from build123d import *

# Parameters (mm, degrees)
F0_W      = 76.2
F0_H      = 76.2
F1_DEPTH  = 76.2
F2_W      = 50.8
F2_H      = 50.8
F3_DEPTH  = 50.8
F4_W      = 7.2508919984
F4_H      = 10.1156122983
F5_DEPTH  = 12.7
F6_R      = 5.08
F7_W      = 8.5941962898
F7_H      = 18.2563401759
F8_DEPTH  = 2.54
F10_W     = 29.7498870641
F10_H     = 30.6668374687
F11_DEPTH = 2.54
F12_R     = 5.08
F13_W     = 35.6998704374
F13_H     = 3.7890225649
F14_DEPTH = 25.4
F16_W     = 13.0332894623
F16_H     = 16.8449506164
F17_DEPTH = 2.54
F18_DEPTH = 2.54
F19_DEPTH = 2.54


with BuildPart() as f1:
    # F0 (on Top) → F1 (new body)
    with BuildSketch(Plane.XY):
        with Locations((-38.1, 38.1)):
            Rectangle(F0_W, F0_H)
    extrude(amount=F1_DEPTH)

    # F2 (on face) → F3 (join)
    with BuildSketch(Plane.YZ):
        with Locations((42.4093476772, 25.4)):
            Rectangle(F2_W, F2_H)
    extrude(amount=F3_DEPTH)

    # F4 (on face) → F5 (join)
    with BuildSketch(Plane.XY.offset(50.8)):
        with Locations((22.3073018715, 41.2539299577)):
            Rectangle(F4_W, F4_H)
    extrude(amount=F5_DEPTH)

    # F6
    f6_edges = [f1.edges().sort_by_distance(p)[0] for p in [
        (22.307302, 36.196124, 63.5),
    ]]
    fillet(f6_edges, radius=F6_R)

    # F7 (on face) → F8 (join)
    with BuildSketch(Plane.XZ):
        with Locations((-42.4338337034, 9.1281700879)):
            Rectangle(F7_W, F7_H)
    extrude(amount=F8_DEPTH)

    # F10 (on face) → F11 (join)
    with BuildSketch(Plane.XZ.offset(-17.0093476772)):
        with Locations((22.7058520541, 15.3334187344)):
            Rectangle(F10_W, F10_H)
    extrude(amount=F11_DEPTH)

    # F12
    f12_edges = [f1.edges().sort_by_distance(p)[0] for p in [
        (-38.1, 0, 76.2),
        (0, 38.1, 76.2),
        (-38.1, 76.2, 76.2),
        (-76.2, 38.1, 76.2),
    ]]
    fillet(f12_edges, radius=F12_R)

    # F13 (on face) → F14 (join)
    with BuildSketch(Plane.XZ):
        with Locations((-39.2985325307, 46.8699112535)):
            Rectangle(F13_W, F13_H)
    extrude(amount=F14_DEPTH)

    # F16 (on face) → F17 (join)
    with BuildSketch(Plane.XZ):
        with Locations((-39.2985325307, 57.1868978441)):
            Rectangle(F16_W, F16_H)
    extrude(amount=F17_DEPTH)

    # F15 (on face) → F18 (join)
    with BuildSketch(Plane.XY.offset(48.7644225359)):
        Polygon((-57.1484677494, -18.2180759441), (-52.4711199105, -25.4), (-48.1553934515, -25.4), (-57.1484677494, -11.2543340924), align=None)
    extrude(amount=F18_DEPTH)

    # F19 (add): a face of the model
    f19_faces = [f1.faces().sort_by_distance(p)[0] for p in [
        (-38.1323314504, -12.5401378745, 48.7644225359),
    ]]
    extrude(f19_faces, amount=F19_DEPTH)


solid = f1.part
For this review, take the finished solid that the model builds, in its own axes (mm). A direction names the side the tool comes from. Round coordinates to 2 decimals unless told otherwise and drop trailing zeros. Order: outer loops, then holes, each group sorted by start corner. A loop starts at its lowest first (then second) coordinate and runs counter-clockwise, first axis right, second up. Notation, with made-up numbers: (86.25, 31) -> (100.25, 31) arc R18 cw to (100.25, 38) -> close; hole circle Ø6 at (-24.75, 10). An arc over 180 degrees is marked (long way). Write item = value, one per line. Start each with the question number.
1) To check wall thickness, follow line 1 (Y direction, x = 14.5, z = 37); line 2 (X direction, y = 55, z = 71); line 3 (Z direction, x = 20.5, y = 61). State the ranges of each line that lie inside material, in increasing order. Write a range as from..to.
2) Insertion check: pin 1 (0.8 mm diameter, centred on y = -0.5, z = 10.5, fed in from +X); pin 2 (1 mm diameter, centred on x = -39.5, z = 39, fed in from -Y); pin 3 (5 mm diameter, centred on x = -55.5, y = -22.5, fed in from +Z); pin 4 (2 mm diameter, centred on x = 27, z = 62.5, fed in from +Y). Each pin has a flat end and moves straight along its axis. Give the tip position at first contact, or say it passes through.
3) Take a section at C-C on z = 23. State the section outline as (x, y) points, plus the area to 3 significant figures.
4) Take a section at D-D on y = 55.5. State the section outline as (x, z) points, plus the area to 3 significant figures.
5) Take a section at A-A on z = 56. State the section outline as (x, y) points, plus the area to 3 significant figures.
6) Tool access review of faces 1 (the face through (-57.148, -13, 48)), 2 (the face through (-42, -2.54, 9)), 3 (the face through (22, 46.312, 57)), 4 (the face through (18.682, 41, 57)), 5 (the face through (22, 44, 63.5)): name each direction out of +Z, -Z, +X, -X, +Y, -Y from which nothing blocks a thin tool from reaching the whole face with its end or side.
7) Take a section at B-B on x = -40. State the section outline as (y, z) points.
Verdict:
q1.line_1 = 17.01..67.81
q1.line_2 = -76.2..0
q1.line_3 = 0..50.8
q2.pin_1 = -38.14
q2.pin_2 = 0
q2.pin_3 = 51.3
q2.pin_4 = through
q3.outline = (-76.2, 0) -> (0, 0) -> (0, 17.01) -> (7.83, 17.01) -> (7.83, 14.47) -> (37.58, 14.47) -> (37.58, 17.01) -> (50.8, 17.01) -> (50.8, 67.81) -> (0, 67.81) -> (0, 76.2) -> (-76.2, 76.2) -> close
q3.area = 8,460 mm2
q4.outline = (-76.2, 0) -> (50.8, 0) -> (50.8, 50.8) -> (0, 50.8) -> (0, 71.12) arc R5.08 ccw to (-5.08, 76.2) -> (-71.12, 76.2) arc R5.08 ccw to (-76.2, 71.12) -> close
q4.area = 8,380 mm2
q5.outline = (-76.2, 0) -> (-45.82, 0) -> (-45.82, -2.54) -> (-32.78, -2.54) -> (-32.78, 0) -> (0, 0) -> (0, 76.2) -> (-76.2, 76.2) -> close; (18.68, 36.2) -> (25.93, 36.2) -> (25.93, 46.31) -> (18.68, 46.31) -> close
q5.area = 5,910 mm2
q6.face_1 = +Z, -Z, -X, -Y
q6.face_2 = -Z, +X, -X, -Y
q6.face_3 = +Z, +X, +Y
q6.face_4 = +Z, +Y, -Y
q6.face_5 = +Z, +X, +Y, -Y
q7.outline = (-25.4, 44.98) -> (0, 44.98) -> (0, 18.26) -> (-2.54, 18.26) -> (-2.54, 0) -> (76.2, 0) -> (76.2, 71.12) arc R5.08 ccw to (71.12, 76.2) -> (5.08, 76.2) arc R5.08 ccw to (0, 71.12) -> (0, 65.61) -> (-2.54, 65.61) -> (-2.54, 51.3) -> (-25.4, 51.3) -> close
